Input: part model. Units: mm. Frame: model coordinates. Face numbers are marked on the shaded views. A direction names the side the tool comes from. Give positions to 0.01 mm unless a question says otherwise; leave off trailing zeros. Write each loop counter-clockwise with the first axis right and the second up, starting at its lowest first coordinate (ties: lowest second). Pieces come first, ordered by that corner, then holes. Notation, with made-up numbers: (22.25, 20) -> (62.25, 20) arc R12 cw to (62.25, 33) -> close; hole circle Ø10 at (89.25, -22). An arc over 180 degrees is marked (long way). Answer as a JSON object with one key per item and string values. Group by question number.
from build123d import *

# Parameters (mm, degrees)
SKETCH1_R           = 31
BOSS_EXTRUDE1_DEPTH = 30
SKETCH1_3_R         = 31
SKETCH1_3_R_2       = 19
BOSS_EXTRUDE2_DEPTH = 20
SKETCH3_W           = 5
SKETCH3_H           = 12
CUT_EXTRUDE7_DEPTH  = 20


with BuildPart() as part:
    # Sketch1 → Boss-Extrude1 (new body)
    with BuildSketch(Plane.XY):
        with BuildLine():
            ThreePointArc((50.448529412, -7.479697868), (43.5, 0), (50.448529412, 7.479697868))
            ThreePointArc((50.448529412, 7.479697868), (50.020049301, 9.949606423), (49.470720222, 12.395476624))
            ThreePointArc((49.470720222, 12.395476624), (40.188759664, 16.646729308), (43.746007316, 26.216156162))
            ThreePointArc((43.746007316, 26.216156162), (42.404950227, 28.334081884), (40.961442331, 30.383552165))
            ThreePointArc((40.961442331, 30.383552165), (30.759144982, 30.759144982), (30.383552165, 40.961442331))
            ThreePointArc((30.383552165, 40.961442331), (28.334081884, 42.404950227), (26.216156162, 43.746007316))
            ThreePointArc((26.216156162, 43.746007316), (16.646729308, 40.188759664), (12.395476624, 49.470720222))
            ThreePointArc((12.395476624, 49.470720222), (9.949606423, 50.020049301), (7.479697868, 50.448529412))
            ThreePointArc((7.479697868, 50.448529412), (0, 43.5), (-7.479697868, 50.448529412))
            ThreePointArc((-7.479697868, 50.448529412), (-9.949606423, 50.020049301), (-12.395476624, 49.470720222))
            ThreePointArc((-12.395476624, 49.470720222), (-16.646729308, 40.188759664), (-26.216156162, 43.746007316))
            ThreePointArc((-26.216156162, 43.746007316), (-28.334081884, 42.404950227), (-30.383552165, 40.961442331))
            ThreePointArc((-30.383552165, 40.961442331), (-30.759144982, 30.759144982), (-40.961442331, 30.383552165))
            ThreePointArc((-40.961442331, 30.383552165), (-42.404950227, 28.334081884), (-43.746007316, 26.216156162))
            ThreePointArc((-43.746007316, 26.216156162), (-40.188759664, 16.646729308), (-49.470720222, 12.395476624))
            ThreePointArc((-49.470720222, 12.395476624), (-50.020049301, 9.949606423), (-50.448529412, 7.479697868))
            ThreePointArc((-50.448529412, 7.479697868), (-43.5, 0), (-50.448529412, -7.479697868))
            ThreePointArc((-50.448529412, -7.479697868), (-50.020049301, -9.949606423), (-49.470720222, -12.395476624))
            ThreePointArc((-49.470720222, -12.395476624), (-40.188759664, -16.646729308), (-43.746007316, -26.216156162))
            ThreePointArc((-43.746007316, -26.216156162), (-42.404950227, -28.334081884), (-40.961442331, -30.383552165))
            ThreePointArc((-40.961442331, -30.383552165), (-30.759144982, -30.759144982), (-30.383552165, -40.961442331))
            ThreePointArc((-30.383552165, -40.961442331), (-28.334081884, -42.404950227), (-26.216156162, -43.746007316))
            ThreePointArc((-26.216156162, -43.746007316), (-16.646729308, -40.188759664), (-12.395476624, -49.470720222))
            ThreePointArc((-12.395476624, -49.470720222), (-9.949606423, -50.020049301), (-7.479697868, -50.448529412))
            ThreePointArc((-7.479697868, -50.448529412), (0, -43.5), (7.479697868, -50.448529412))
            ThreePointArc((7.479697868, -50.448529412), (9.949606423, -50.020049301), (12.395476624, -49.470720222))
            ThreePointArc((12.395476624, -49.470720222), (16.646729308, -40.188759664), (26.216156162, -43.746007316))
            ThreePointArc((26.216156162, -43.746007316), (28.334081884, -42.404950227), (30.383552165, -40.961442331))
            ThreePointArc((30.383552165, -40.961442331), (30.759144982, -30.759144982), (40.961442331, -30.383552165))
            ThreePointArc((40.961442331, -30.383552165), (42.404950227, -28.334081884), (43.746007316, -26.216156162))
            ThreePointArc((43.746007316, -26.216156162), (40.188759664, -16.646729308), (49.470720222, -12.395476624))
            ThreePointArc((49.470720222, -12.395476624), (50.020049301, -9.949606423), (50.448529412, -7.479697868))
        make_face()
        Circle(SKETCH1_R, mode=Mode.SUBTRACT)
    extrude(amount=BOSS_EXTRUDE1_DEPTH)

    # Sketch1<3> → Boss-Extrude2 (add)
    with BuildSketch(Plane.XY):
        Circle(SKETCH1_3_R)
        Circle(SKETCH1_3_R_2, mode=Mode.SUBTRACT)
    extrude(amount=BOSS_EXTRUDE2_DEPTH)

    # Sketch3 → Cut-Extrude7 (cut)
    with BuildSketch(Plane.XY):
        with Locations((0, 18.767120851)):
            Rectangle(SKETCH3_W, SKETCH3_H)
    extrude(amount=CUT_EXTRUDE7_DEPTH, mode=Mode.SUBTRACT)


solid = part.part
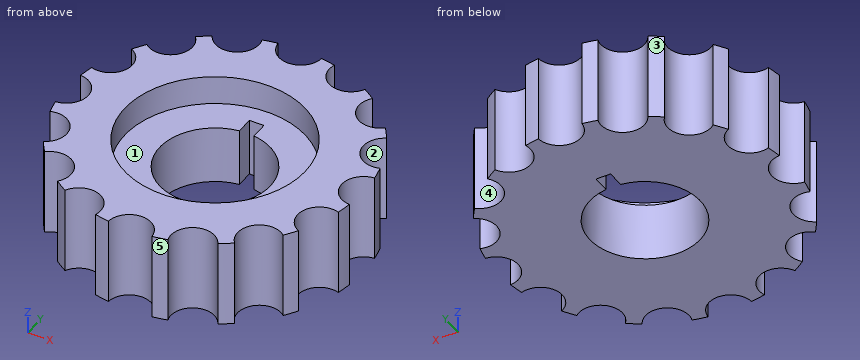
1. Mould query, pull axis Y, two halves, no side actions, for the marked faces 3, 4 and 5. Classes: pulls with the +Y half, pulls with the -Y half, needs draft (parallel to the pull), parting line crosses it, or undercut.
2. Section B-B (x = -15). Return the cut outline in (y, z).
3. Contact query for flat-ended pins moving along their axis: pin 1 Ø6 at (y, z) = (-11, 7.5) entering from +X; pin 2 Ø4.5 at (y, z) = (22.5, 9.5) entering from +X; pin 3 Ø12 at (y, z) = (22, 12.5) entering from -X. Output: stop coordinate, or through.
4. Line query: line 1 (Y direction, x = 10, z = 14); line 2 (Y direction, x = 16, z = 10.5); line 3 (Z direction, x = -1, y = 29). Output: solid intervals per line, ascending.
5. Reachability of the marked faces 1 and 2 from +Z, -Z, +X, -X, +Y, -Y: full face, straight path, thin tool, end or side. Return the list, or none.
6. Section C-C (y = 0). Return the cut outline in (x, z), plus the area to 3 significant figures.
Working result:
{
 "1": {"face 3": "pulls with the +Y half", "face 4": "undercut", "face 5": "pulls with the -Y half"},
 "2": {"outline": "(-41.13, 0) -> (-11.66, 0) -> (-11.66, 20) -> (-27.13, 20) -> (-27.13, 30) -> (-41.13, 30) -> close; (11.66, 0) -> (41.13, 0) -> (41.13, 30) -> (27.13, 30) -> (27.13, 20) -> (11.66, 20) -> close"},
 "3": {"pin 1": "stops at x = 50.37", "pin 2": "stops at x = 41.75", "pin 3": "stops at x = -43.75"},
 "4": {"line 1": "y = -50.01 to -16.16, 16.16 to 50.01", "line 2": "y = -40.49 to -10.25, 10.25 to 40.49", "line 3": "z = 0 to 20"},
 "5": {"face 1": "+Z", "face 2": "+Z, -Z"},
 "6": {"outline": "(-43.5, 0) -> (-19, 0) -> (-19, 20) -> (-31, 20) -> (-31, 30) -> (-43.5, 30) -> close; (19, 0) -> (43.5, 0) -> (43.5, 30) -> (31, 30) -> (31, 20) -> (19, 20) -> close", "area": "1,230 mm^2"}
}
